For this review, take the finished solid that the model builds, in its own axes (mm). A direction names the side the tool comes from. Coordinates: 2 decimals unless noted, no trailing zeros. Loops run counter-clockwise (first coordinate to the right, second up) from the corner with the lowest first, then second, coordinate; pieces in that order, holes last. Notation, with made-up numbers: (-4.75, 24) -> (10.25, 24) arc R16 cw to (10.25, 31) -> close; hole circle Ø11 at (-13.75, -4). An arc over 180 degrees is marked (long way). Use a Markdown table: item, result.
from build123d import *

# Parameters (mm, degrees)
SKETCH3_W               = 116
SKETCH3_H               = 416
BOSS_EXTRUDE1_DEPTH     = 10
SKETCH4_W               = 100
SKETCH4_H               = 400
CUT_EXTRUDE1_DEPTH      = 8
SKETCH6_W               = 3
SKETCH6_H               = 100
BOSS_EXTRUDE4_DEPTH     = 3
SKETCH7_R               = 1.5
BOSS_EXTRUDE5_DEPTH     = 3
CUT_EXTRUDE3_DEPTH      = 10
CUT_EXTRUDE3_DEPTH_BACK = 10
SKETCH8_W               = 116
SKETCH8_H               = 200
CUT_EXTRUDE4_DEPTH      = 10
SKETCH11_W              = 8
SKETCH11_H              = 16
CUT_EXTRUDE5_DEPTH      = 10
SKETCH13_R              = 1.5
BOSS_EXTRUDE8_DEPTH     = 3


with BuildPart() as part:
    # Sketch3 → Boss-Extrude1 (new body)
    with BuildSketch(Plane(origin=(0, 0, 0), x_dir=(1, 0, 0), z_dir=(0, 1, 0))):
        with Locations((-1098.104867157, 569.267379684)):
            Rectangle(SKETCH3_W, SKETCH3_H)
    extrude(amount=BOSS_EXTRUDE1_DEPTH)

    # Sketch4 → Cut-Extrude1 (cut)
    with BuildSketch(Plane(origin=(0, 10, 0), x_dir=(1, 0, 0), z_dir=(0, 1, 0))):
        with Locations((-1098.104867157, 569.267379684)):
            Rectangle(SKETCH4_W, SKETCH4_H)
    extrude(amount=-CUT_EXTRUDE1_DEPTH, mode=Mode.SUBTRACT)

    # Sketch6 → Boss-Extrude4 (add)
    with BuildSketch(Plane(origin=(0, 2, 0), x_dir=(1, 0, 0), z_dir=(0, 1, 0))):
        with Locations((-1129.604867157, 719.267379684)):
            Rectangle(SKETCH6_W, SKETCH6_H)
        with Locations((-1066.604867157, 719.267379684)):
            Rectangle(SKETCH6_W, SKETCH6_H)
    extrude(amount=BOSS_EXTRUDE4_DEPTH)

    # Sketch7 → Boss-Extrude5 (add)
    with BuildSketch(Plane(origin=(0, 2, 0), x_dir=(1, 0, 0), z_dir=(0, 1, 0))):
        with Locations(Location((-1085.404867157, 452.168271652, 0), (0, 0, 270))):
            Circle(SKETCH7_R)
    extrude(amount=BOSS_EXTRUDE5_DEPTH)

    # Sketch8 → Cut-Extrude3 (cut, two sides: drawn at the far end of the back side and taken through both)
    with BuildSketch(Plane(origin=(0, 2, 0), x_dir=(1, 0, 0), z_dir=(0, 1, 0)).offset(-CUT_EXTRUDE3_DEPTH_BACK)):
        with Locations((-1098.104867157, 677.267379684)):
            Rectangle(SKETCH8_W, SKETCH8_H)
    extrude(amount=CUT_EXTRUDE3_DEPTH + CUT_EXTRUDE3_DEPTH_BACK, mode=Mode.SUBTRACT)

    # Sketch9 → Cut-Extrude4 (cut)
    with BuildSketch(Plane(origin=(0, 2, 0), x_dir=(1, 0, 0), z_dir=(0, 1, 0))):
        Polygon((-1156.104867157, 577.267379684), (-1156.104867157, 561.267379684), (-1127.104867157, 561.267379684), (-1127.104867157, 571.267379684), (-1132.104867157, 571.267379684), (-1132.104867157, 577.267379684), align=None)
        Polygon((-1079.104867157, 577.267379684), (-1117.104867157, 577.267379684), (-1117.104867157, 571.267379684), (-1122.104867157, 571.267379684), (-1122.104867157, 561.267379684), (-1074.104867157, 561.267379684), (-1074.104867157, 571.267379684), (-1079.104867157, 571.267379684), align=None)
        Polygon((-1069.104867157, 561.267379684), (-1048.104867157, 561.267379684), (-1048.104867157, 577.267379684), (-1064.104867157, 577.267379684), (-1064.104867157, 571.267379684), (-1069.104867157, 571.267379684), align=None)
    extrude(amount=-CUT_EXTRUDE4_DEPTH, mode=Mode.SUBTRACT)

    # Sketch11 → Cut-Extrude5 (cut)
    with BuildSketch(Plane(origin=(0, 10, 0), x_dir=(1, 0, 0), z_dir=(0, 1, 0))):
        with Locations((-1152.104867157, 569.267379684)):
            Rectangle(SKETCH11_W, SKETCH11_H)
        with Locations((-1044.104867157, 569.267379684)):
            Rectangle(SKETCH11_W, SKETCH11_H)
    extrude(amount=-CUT_EXTRUDE5_DEPTH, mode=Mode.SUBTRACT)

    # Sketch13 → Boss-Extrude8 (add)
    with BuildSketch(Plane(origin=(0, 2, 0), x_dir=(1, 0, 0), z_dir=(0, 1, 0))):
        with Locations(Location((-1110.804867157, 452.168271652, 0), (0, 0, 270))):
            Circle(SKETCH13_R)
    extrude(amount=BOSS_EXTRUDE8_DEPTH)


solid = part.part
(1) Take a section at D-D on x = -1105. Write out the cut boundary in (y, z).
Found:
| item | result |
|---|---|
| outline | (0, -561.27) -> (2, -561.27) -> (2, -369.27) -> (10, -369.27) -> (10, -361.27) -> (0, -361.27) -> close |
(2) Take a section at C-C on y = 7.5. Write out the cut boundary in (x, z), plus the area to 3 significant figures.
Found:
| item | result |
|---|---|
| outline | (-1156.1, -561.27) -> (-1148.1, -561.27) -> (-1148.1, -369.27) -> (-1048.1, -369.27) -> (-1048.1, -561.27) -> (-1040.1, -561.27) -> (-1040.1, -361.27) -> (-1156.1, -361.27) -> close |
| area | 4,000 mm^2 |
(3) Take a section at A-A on x = -1076.5. Write out the cut boundary in (y, z).
Found:
| item | result |
|---|---|
| outline | (0, -577.27) -> (2, -577.27) -> (2, -571.27) -> (0, -571.27) -> close; (0, -561.27) -> (2, -561.27) -> (2, -369.27) -> (10, -369.27) -> (10, -361.27) -> (0, -361.27) -> close |
(4) For faces 1 (the face through (-1040.105, 5, -460)), 2 (the face through (-1048.105, 6, -464)), 3 (the face through (-1048.4, 1.7, -561.267)), list the 3-axis set-ups (+Z, -Z, +X, -X, +Y, -Y) from which the entire face can be reached by the end or side of a thin tool; tool diameter is ignored.
Found:
| item | result |
|---|---|
| face 1 | +Z, -Z, +X, +Y, -Y |
| face 2 | -Z, +Y |
| face 3 | +X, +Y, -Y |
(5) For pin 1 Ø4 at (x, y) = (-1114.5, 5) entering from -Z; pin 2 Ø2 at (y, z) = (0.5, -564.5) entering from -X; pin 3 Ø0.6 at (x, y) = (-1090.5, 0.5) entering from -Z, all flat-tipped, find the tip position at first contact; note any pin that passes through.
Found:
| item | result |
|---|---|
| pin 1 | stops at z = -369.27 |
| pin 2 | stops at x = -1127.1 |
| pin 3 | stops at z = -561.27 |
(6) Take a section at B-B on z = -428.5. Write out the cut boundary in (x, y).
Found:
| item | result |
|---|---|
| outline | (-1156.1, 0) -> (-1040.1, 0) -> (-1040.1, 10) -> (-1048.1, 10) -> (-1048.1, 2) -> (-1148.1, 2) -> (-1148.1, 10) -> (-1156.1, 10) -> close |
(7) For line 1 along X through (y, z) = (7.25, -466.5); line 2 along Y through (x, z) = (-1112.5, -513.5); line 3 along Z through (x, y) = (-1139, 2.25), list the stretches that pass through material, from the lowest coordinate up.
Found:
| item | result |
|---|---|
| line 1 | x = -1156.1 to -1148.1, -1048.1 to -1040.1 |
| line 2 | y = 0 to 2 |
| line 3 | z = -369.27 to -361.27 |
(8) Mouldability with a two-part tool opening along X and no side actions: class faces 4 (the face through (-1148.105, 6, -464)), 5 (the face through (-1156.105, 5, -460)), 6 (the face through (-1099, 0, -471)) as pulls with the +X half, pulls with the -X half, needs draft (parallel to the pull), parting line crosses it, or undercut.
Found:
| item | result |
|---|---|
| face 4 | undercut |
| face 5 | pulls with the -X half |
| face 6 | needs draft |
